The drawing under review shows one solid part. Ordinate dimensions are in mm from its lowest x, y, z. A direction names the side the tool comes from. Coordinates: 2 decimals unless noted, no trailing zeros. Order: outer loops, then holes, each group sorted by start corner. A loop starts at its lowest first (then second) coordinate and runs counter-clockwise, first axis right, second up. Notation, with made-up numbers: (69, 1.5) -> (128, 1.5) arc R11 ccw to (128, 7.5) -> close; hole circle Ø10 at (-11.5, 59.25). An arc over 180 degrees is marked (long way). Write item = value, one per line.
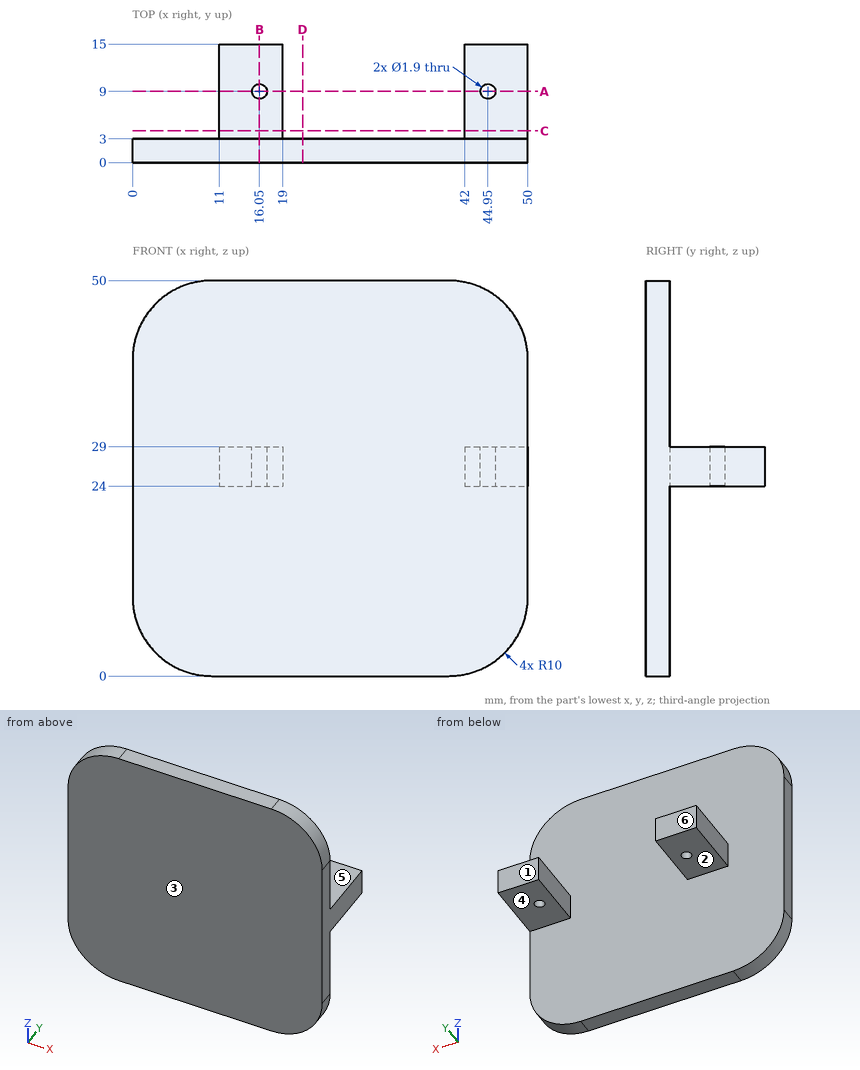
(1) We need section A-A (y = 9). Write out the cut boundary in (x, z), and give its area (3 significant figures).
Report:
outline = (11, 24) -> (15.1, 24) -> (15.1, 29) -> (11, 29) -> close; (17, 24) -> (19, 24) -> (19, 29) -> (17, 29) -> close; (42, 24) -> (44, 24) -> (44, 29) -> (42, 29) -> close; (45.9, 24) -> (50, 24) -> (50, 29) -> (45.9, 29) -> close
area = 61.0 mm²
(2) We need section B-B (x = 16.05). Write out the cut boundary in (y, z), and give its area (4 significant figures).
Report:
outline = (0, 0) -> (3, 0) -> (3, 24) -> (8.05, 24) -> (8.05, 29) -> (3, 29) -> (3, 50) -> (0, 50) -> close; (9.95, 24) -> (15, 24) -> (15, 29) -> (9.95, 29) -> close
area = 200.5 mm²
(3) Insertion check: pin 1 (3 mm diameter, centred on x = 12.5, z = 43.5, fed in from +Y); pin 2 (4 mm diameter, centred on x = 14, y = 9.5, fed in from +Z); pin 3 (2.5 mm diameter, centred on y = 10.5, z = 25.5, fed in from -X). Each pin has a flat end and moves straight along its axis. Give the tip position at first contact, or say it passes through.
Report:
pin_1 = 3
pin_2 = 29
pin_3 = 11
(4) For L1, parallel to Y at x = 44.95, z = 27.6; L2, parallel to X at y = 5.75, z = 26; L3, parallel to Z at x = 12.5, y = 4.25, list the stretches that pass through material, from the lowest coordinate up.
Report:
L1 = 0 to 8.05, 9.95 to 15
L2 = 11 to 19, 42 to 50
L3 = 24 to 29
(5) The part is to be moulded in two halves that separate along Y. For the marked faces 1, 2 and 3, say which applies: released by +Y, released by -Y, zero draft, split by the parting line, or undercut.
Report:
face_1 = released by +Y
face_2 = zero draft
face_3 = released by -Y
(6) We need section D-D (x = 21.5). Write out the cut boundary in (y, z), and give its area (3 significant figures).
Report:
outline = (0, 0) -> (3, 0) -> (3, 50) -> (0, 50) -> close
area = 150 mm²
(7) For the marked faces 4, 5 and 6, list the 3-axis set-ups (+Z, -Z, +X, -X, +Y, -Y) from which the entire face can be reached by the end or side of a thin tool; tool diameter is ignored.
Report:
face_4 = -Z, +X, -X, +Y
face_5 = +Z, +X, -X, +Y
face_6 = +Z, -Z, +X, -X, +Y
(8) We need section C-C (y = 4). Write out the cut boundary in (x, z).
Report:
outline = (11, 24) -> (19, 24) -> (19, 29) -> (11, 29) -> close; (42, 24) -> (50, 24) -> (50, 29) -> (42, 29) -> close
